For this review, take the finished solid that the model builds, in its own axes (mm). A direction names the side the tool comes from. Round coordinates to 2 decimals unless told otherwise and drop trailing zeros. Order: outer loops, then holes, each group sorted by start corner. A loop starts at its lowest first (then second) coordinate and runs counter-clockwise, first axis right, second up. Notation, with made-up numbers: (29.5, -22) - (84.5, -22) arc R23 ccw to (84.5, 16) - close; hole circle Ø5 at (69.5, 31.5). An arc over 180 degrees is marked (long way). One line per question, with ' | ' between items.
```python
from build123d import *

# Parameters (mm, degrees)
ENL_V_START             = -0.5
ENL_V_MAT_EXTRU_1_DEPTH = 10


with BuildPart() as part:
    # Esquisse1 → Révolution1 (revolve)
    with BuildSketch(Plane.XY):
        with BuildLine():
            Line((2.5, 68), (1.5, 68))
            Line((1.5, 68), (1.5, 0))
            Line((1.5, 0), (0, 0))
            Line((0, 0), (0, 70))
            ThreePointArc((0, 70), (1.600781059, 69.438476324), (2.5, 68))
        make_face()
    revolve(axis=Axis((0, 0, 0), (0, 1, 0)))

    # Esquisse2 → Enlèv. mat.-Extru.1 (cut)
    with BuildSketch(Plane.XZ.offset(-68).offset(ENL_V_START)):
        with BuildLine():
            Line((2.5, 1), (-4.803104299, 1))
            ThreePointArc((-4.803104299, 1), (-5.803104299, 0), (-4.803104299, -1))
            Line((-4.803104299, -1), (2.5, -1))
            ThreePointArc((2.5, -1), (3.5, 0), (2.5, 1))
        make_face()
    extrude(amount=-ENL_V_MAT_EXTRU_1_DEPTH, mode=Mode.SUBTRACT)


solid = part.part
```
(1) For faces 4 (the flat face through (0, 68, 2)), 5 (the flat face through (0, 68.5, 0)), list the 3-axis set-ups (+Z, -Z, +X, -X, +Y, -Y) from which the entire face can be reached by the end or side of a thin tool; tool diameter is ignored.
Output values:
face 4: -Y | face 5: +X, -X, +Y
(2) Insertion check: pin 1 (1 mm diameter, centred on x = 0.5, y = 69.5, fed in from +Z); pin 2 (2 mm diameter, centred on y = 25, z = 0, fed in from -X); pin 3 (0.6 mm diameter, centred on x = 0, y = 69.5, fed in from -Z). Each pin has a flat end and moves straight along its axis. Give the tip position at first contact, or say it passes through.
Output values:
pin 1: z = 1.98 | pin 2: x = -1.5 | pin 3: z = -1.86
(3) We need section B-B on z = 0. State the section outline as (x, y) points (1 decimal), plus the area to 3 significant figures.
Output values:
outline: (-2.5, 68) - (-1.5, 68) - (-1.5, 0) - (1.5, 0) - (1.5, 68) - (2.5, 68) arc R2.6 ccw to (2.3, 68.5) - (-2.3, 68.5) arc R2.6 ccw to start | area: 206 mm^2
(4) We need section A-A on x = 0. State the section outline as (y, z) points (1 decimal), plus the area to 3 significant figures.
Output values:
outline: (0, -1.5) - (68, -1.5) - (68, -2.5) arc R2.6 ccw to (69.8, -1) - (68.5, -1) - (68.5, 1) - (69.8, 1) arc R2.6 ccw to (68, 2.5) - (68, 1.5) - (0, 1.5) - close | area: 209 mm^2
(5) We need section C-C on y = 15. State the section outline as (x, z) points, plus the area to 3 significant figures.
Output values:
outline: circle Ø3 at (0, 0) | area: 7.07 mm^2
(6) For probe 1 along Y at (x, z) = (-1.7, 0.95); probe 2 along Z at (x, y) = (0.05, 3); probe 3 along X at (y, z) = (10.5, -0.15), list the stretches that pass through material, from the lowest coordinate up. Write a range as [from, to].
Output values:
probe 1: [68, 68.5] | probe 2: [-1.5, 1.5] | probe 3: [-1.49, 1.49]
(7) Mouldability with a two-part tool opening along Z and no side actions: class faces 1 (the flat face through (0, 69, -1)), 2 (the cylindrical face through (-1.5, 33.52, -0.07)), 3 (the flat face through (0, 0, 0)) as released by +Z, released by -Z, zero draft, split by the parting line, or undercut.
Output values:
face 1: undercut | face 2: split by the parting line | face 3: zero draft
